from build123d import *

# Parameters (mm, degrees)
BOSS_EXTRUDE1_DEPTH = 20
CUT_EXTRUDE1_DEPTH  = 188.710441905
BOSS_EXTRUDE2_DEPTH = 2
SKETCH4_W           = 9
SKETCH4_H           = 4.5
CUT_EXTRUDE2_DEPTH  = 185.20565812
SKETCH5_R           = 1
CUT_EXTRUDE3_DEPTH  = 185.20565812


with BuildPart() as part:
    # Sketch1 → Boss-Extrude1 (new body)
    with BuildSketch(Plane.XY):
        with BuildLine():
            Line((-153.675, 0.1), (-153.675, 90.1))
            ThreePointArc((-153.675, 90.1), (-151.917640687, 94.342640687), (-147.675, 96.1))
            Line((-147.675, 96.1), (0.325, 96.1))
            ThreePointArc((0.325, 96.1), (4.567640687, 94.342640687), (6.325, 90.1))
            Line((6.325, 90.1), (6.325, 0.1))
            ThreePointArc((6.325, 0.1), (4.567640687, -4.142640687), (0.325, -5.9))
            Line((0.325, -5.9), (-147.675, -5.9))
            ThreePointArc((-147.675, -5.9), (-151.917640687, -4.142640687), (-153.675, 0.1))
        make_face()
        with BuildLine():
            Line((3.325, 90.1), (3.325, 0.1))
            ThreePointArc((3.325, 0.1), (2.446320344, -2.021320344), (0.325, -2.9))
            Line((0.325, -2.9), (-147.675, -2.9))
            ThreePointArc((-147.675, -2.9), (-149.796320344, -2.021320344), (-150.675, 0.1))
            Line((-150.675, 0.1), (-150.675, 90.1))
            ThreePointArc((-150.675, 90.1), (-149.796320344, 92.221320344), (-147.675, 93.1))
            Line((-147.675, 93.1), (0.325, 93.1))
            ThreePointArc((0.325, 93.1), (2.446320344, 92.221320344), (3.325, 90.1))
        make_face(mode=Mode.SUBTRACT)
    extrude(amount=BOSS_EXTRUDE1_DEPTH)

    # Sketch2 → Cut-Extrude1 (cut, through all)
    with BuildSketch(Plane(origin=(6.325, 0, 0), x_dir=(0, 0, -1), z_dir=(1, 0, 0))):
        Polygon((-20, 96.1), (-12, 96.1), (-20, -5.9), align=None)
    extrude(amount=-CUT_EXTRUDE1_DEPTH, mode=Mode.SUBTRACT)

    # Sketch3 → Boss-Extrude2 (add)
    with BuildSketch(Plane(origin=(0, 1.522965227, 19.417806649), x_dir=(1, 0, 0), z_dir=(0, 0.0781912453186315, 0.9969383778125516))):
        with BuildLine():
            Line((-153.675, 88.849057017), (-153.675, -1.427335188))
            add(Edge.make_bspline(
                [(-153.675, -1.427335188), (-153.675, -7.445761335), (-147.675, -7.445761335)],
                knots=[1.570796327, 1.570796327, 1.570796327, 3.141592654, 3.141592654, 3.141592654], degree=2, weights=[1, 0.707106781, 1]))
            Line((-147.675, -7.445761335), (0.325, -7.445761335))
            add(Edge.make_bspline(
                [(0.325, -7.445761335), (6.325, -7.445761335), (6.325, -1.427335188)],
                knots=[3.141592654, 3.141592654, 3.141592654, 4.71238898, 4.71238898, 4.71238898], degree=2, weights=[1, 0.707106781, 1]))
            Line((6.325, -1.427335188), (6.325, 88.849057017))
            add(Edge.make_bspline(
                [(6.325, 88.849057017), (6.325, 94.867483164), (0.325, 94.867483164)],
                knots=[4.71238898, 4.71238898, 4.71238898, 6.283185307, 6.283185307, 6.283185307], degree=2, weights=[1, 0.707106781, 1]))
            Line((0.325, 94.867483164), (-147.675, 94.867483164))
            add(Edge.make_bspline(
                [(-147.675, 94.867483164), (-153.675, 94.867483164), (-153.675, 88.849057017)],
                knots=[0, 0, 0, 1.570796327, 1.570796327, 1.570796327], degree=2, weights=[1, 0.707106781, 1]))
        make_face()
    extrude(amount=BOSS_EXTRUDE2_DEPTH)

    # Sketch4 → Cut-Extrude2 (cut, through all)
    with BuildSketch(Plane(origin=(0, -2.9, 0), x_dir=(1, 0, 0), z_dir=(0, 1, 0))):
        with Locations((-131.175, -10.25)):
            Rectangle(SKETCH4_W, SKETCH4_H)
    extrude(amount=-CUT_EXTRUDE2_DEPTH, mode=Mode.SUBTRACT)

    # Sketch5 → Cut-Extrude3 (cut, through all)
    with BuildSketch(Plane(origin=(0, -2.9, 0), x_dir=(1, 0, 0), z_dir=(0, 1, 0))):
        with Locations(Location((-5.675, -10.25, 0), (0, 0, 180))):
            Circle(SKETCH5_R)
        with Locations(Location((-9.675, -10.25, 0), (0, 0, 180))):
            Circle(SKETCH5_R)
    extrude(amount=-CUT_EXTRUDE3_DEPTH, mode=Mode.SUBTRACT)


solid = part.part
The model under review builds one solid part; all positions refer to its coordinate system, in mm. A direction names the side the tool comes from. Give positions to 0.01 mm unless a question says otherwise; leave off trailing zeros. Order: outer loops, then holes, each group sorted by start corner. A loop starts at its lowest first (then second) coordinate and runs counter-clockwise, first axis right, second up. Notation, with made-up numbers: M 84.5,-35.75 L 122.5,-35.75 A19 cw 122.5,-11.75 Z; hole C 61,63 d3. An arc over 180 degrees is marked long. Use one line per item in the form item = value. Start each with the question number.
Item 1: We need section C-C on y = 58.5. Give the boundary of the cut face in (x, z) (3 decimals), plus the area to 3 significant figures.
Item 2: We need section D-D on y = 21.5. Give the boundary of the cut face in (x, z) (3 decimals).
Item 3: Insertion check: pin 1 Ø8 at (x, y) = (-27.5, 16.5) entering from -Z; pin 2 Ø12 at (x, y) = (-15.5, 57.5) entering from -Z; pin 3 Ø13 at (x, z) = (-43.5, 4) entering from +Y. Each pin has a flat end and moves straight along its axis. Give the tip position at first contact, or say it passes through.
Item 4: We need section B-B on x = -60. Give the boundary of the cut face in (y, z), plus the area to 3 significant figures.
Item 5: For faces 5 (the flat face through (-126.675, -4, 10)), 6 (the flat face through (-75, 96.1, 6)), 7 (the flat face through (-73, -2.9, 10)), 8 (the cylindrical face through (4.52, 94.39, 6.15)), list the 3-axis set-ups (+Z, -Z, +X, -X, +Y, -Y) from which the entire face can be reached by the end or side of a thin tool; tool diameter is ignored.
Item 6: The part is to be moulded in two halves that separate along X. For faces 1 (the flat face through (6.325, 44, 10)), 2 (the flat face through (-75, 93.1, 6)), 3 (the cylindrical face through (-151.96, 94.3, 6.15)), 4 (the cylindrical face through (2.47, -2, 9.74)), say which applies: pulls with the +X half, pulls with the -X half, needs draft (parallel to the pull), parting line crosses it, or undercut.
Item 7: To check wall thickness, follow line 1 along Y through (x, z) = (-102, 1); line 2 along X through (y, z) = (71, 13) (3 decimals); line 3 along Z through (x, y) = (-98, 0). State the ranges of each line that lie inside material, in increasing order. Write a range as from..to.
Item 8: We need section A-A on z = 4.5. Give the boundary of the cut face in (x, y) (3 decimals), plus the area to 3 significant figures.
Completed:
q1.outline = M -153.675,0 L -150.675,0 L -150.675,14.949 L 3.325,14.949 L 3.325,0 L 6.325,0 L 6.325,16.955 L -153.675,16.955 Z
q1.area = 411 mm²
q2.outline = M -153.675,0 L -150.675,0 L -150.675,17.851 L 3.325,17.851 L 3.325,0 L 6.325,0 L 6.325,19.857 L -153.675,19.857 Z
q3.pin_1 = 17.93
q3.pin_2 = 14.56
q3.pin_3 = 96.1
q4.outline = M -5.9,0 L -2.9,0 L -2.9,19.76 L 93.1,12.24 L 93.1,0 L 96.1,0 L 96.1,12 L 96.26,13.99 L -5.74,21.99 L -5.9,20 Z
q4.area = 301 mm²
q5.face_5 = -Y
q5.face_6 = -Z, +X, -X, +Y
q5.face_7 = -Z
q5.face_8 = -Z, +X, +Y
q6.face_1 = pulls with the +X half
q6.face_2 = undercut
q6.face_3 = pulls with the -X half
q6.face_4 = undercut
q7.line_1 = -5.9..-2.9, 93.1..96.1
q7.line_2 = -153.675..-150.675, 3.325..6.325
q7.line_3 = 19.54..21.54
q8.outline = M -153.675,0.1 A6 ccw -147.675,-5.9 L 0.325,-5.9 A6 ccw 6.325,0.1 L 6.325,90.1 A6 ccw 0.325,96.1 L -147.675,96.1 A6 ccw -153.675,90.1 Z; hole M -150.675,0.1 A3 ccw -147.675,-2.9 L 0.325,-2.9 A3 ccw 3.325,0.1 L 3.325,90.1 A3 ccw 0.325,93.1 L -147.675,93.1 A3 ccw -150.675,90.1 Z
q8.area = 1,510 mm²
